The model under review builds one solid part; all positions refer to its coordinate system, in mm. Round coordinates to 2 decimals unless told otherwise and drop trailing zeros. Order: outer loops, then holes, each group sorted by start corner. A loop starts at its lowest first (then second) coordinate and runs counter-clockwise, first axis right, second up.
from build123d import *

# Parameters (mm, degrees)
SKETCH_1_R      = 1.75
SKETCH_1_R_2    = 3.05
EXTRUDE_1_DEPTH = 2


with BuildPart() as part:
    # 草图1 → 凸台-拉伸1 (new body)
    with BuildSketch(Plane(origin=(0, 0, 0), x_dir=(1, 0, 0), z_dir=(0, 1, 0))):
        with BuildLine():
            ThreePointArc((11.700960917, 17.23545404), (5.956293754, 15.563872091), (0, 15))
            Line((0, 15), (-3, 15))
            ThreePointArc((-3, 15), (-4.414213562, 14.414213562), (-5, 13))
            Line((-5, 13), (-5, 2))
            ThreePointArc((-5, 2), (-4.414213562, 0.585786438), (-3, 0))
            Line((-3, 0), (33, 0))
            ThreePointArc((33, 0), (34.414213562, 0.585786438), (35, 2))
            Line((35, 2), (35, 13))
            ThreePointArc((35, 13), (34.414213562, 14.414213562), (33, 15))
            Line((33, 15), (30, 15))
            ThreePointArc((30, 15), (24.043706246, 15.563872091), (18.299039083, 17.23545404))
            ThreePointArc((18.299039083, 17.23545404), (15, 18), (11.700960917, 17.23545404))
        make_face()
        with Locations(Location((30, 7.5, 0), (0, 0, 270))):
            Circle(SKETCH_1_R, mode=Mode.SUBTRACT)
        with Locations(Location((0, 7.5, 0), (0, 0, 270))):
            Circle(SKETCH_1_R, mode=Mode.SUBTRACT)
        with Locations(Location((15, 10.5, 0), (0, 0, 270))):
            Circle(SKETCH_1_R_2, mode=Mode.SUBTRACT)
    extrude(amount=EXTRUDE_1_DEPTH)


solid = part.part
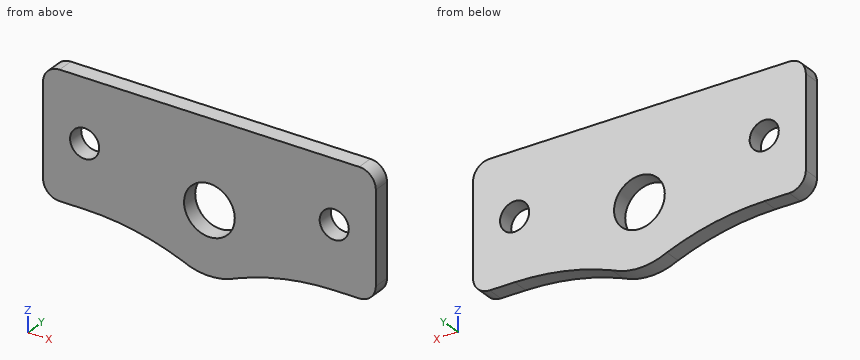
(1) Clearance check with a flat-ended pin moving along its axis: P1, Ø2, axis at x = 0, z = -7.5, coming from the +Y side. State where the tip first meets the part, or that it passes through.
(2) To check wall thickness, follow L1, parallel to X at y = 0.95, z = -10.5; L2, parallel to X at y = 1.4, z = -8.5; L3, parallel to X at y = 0.5, z = -11.75. State the ranges of each line that lie inside material, in increasing order.
(3) We need section C-C (y = 0.75). Give the boundary of the cut face in (x, z), and give its area (3 significant figures).
(4) We need section D-D (z = -8.25). Give the boundary of the cut face in (x, y), and give its area (3 significant figures).
(5) We need section B-B (x = 15). Give the boundary of the cut face in (y, z).
(6) We need section A-A (z = -10.5). Give the boundary of the cut face in (x, y).
Verdict:
1. P1: passes through
2. L1: x = -5 to 11.95, 18.05 to 35
2. L2: x = -5 to -1.44, 1.44 to 12.7, 17.3 to 28.56, 31.44 to 35
2. L3: x = -5 to 12.22, 17.78 to 35
3. outline: (-5, -13) arc R2 ccw to (-3, -15) - (0, -15) arc R31.74 cw to (11.7, -17.24) arc R7.5 ccw to (18.3, -17.24) arc R31.74 cw to (30, -15) - (33, -15) arc R2 ccw to (35, -13) - (35, -2) arc R2 ccw to (33, 0) - (-3, 0) arc R2 ccw to (-5, -2) - close; hole circle Ø3.5 at (0, -7.5); hole circle Ø6.1 at (15, -10.5); hole circle Ø3.5 at (30, -7.5)
3. area: 583 mm2
4. outline: (-5, 0) - (-1.58, 0) - (-1.58, 2) - (-5, 2) - close; (1.58, 0) - (12.94, 0) - (12.94, 2) - (1.58, 2) - close; (17.06, 0) - (28.42, 0) - (28.42, 2) - (17.06, 2) - close; (31.58, 0) - (35, 0) - (35, 2) - (31.58, 2) - close
4. area: 59.1 mm2
5. outline: (0, -18) - (2, -18) - (2, -13.55) - (0, -13.55) - close; (0, -7.45) - (2, -7.45) - (2, 0) - (0, 0) - close
6. outline: (-5, 0) - (11.95, 0) - (11.95, 2) - (-5, 2) - close; (18.05, 0) - (35, 0) - (35, 2) - (18.05, 2) - close
